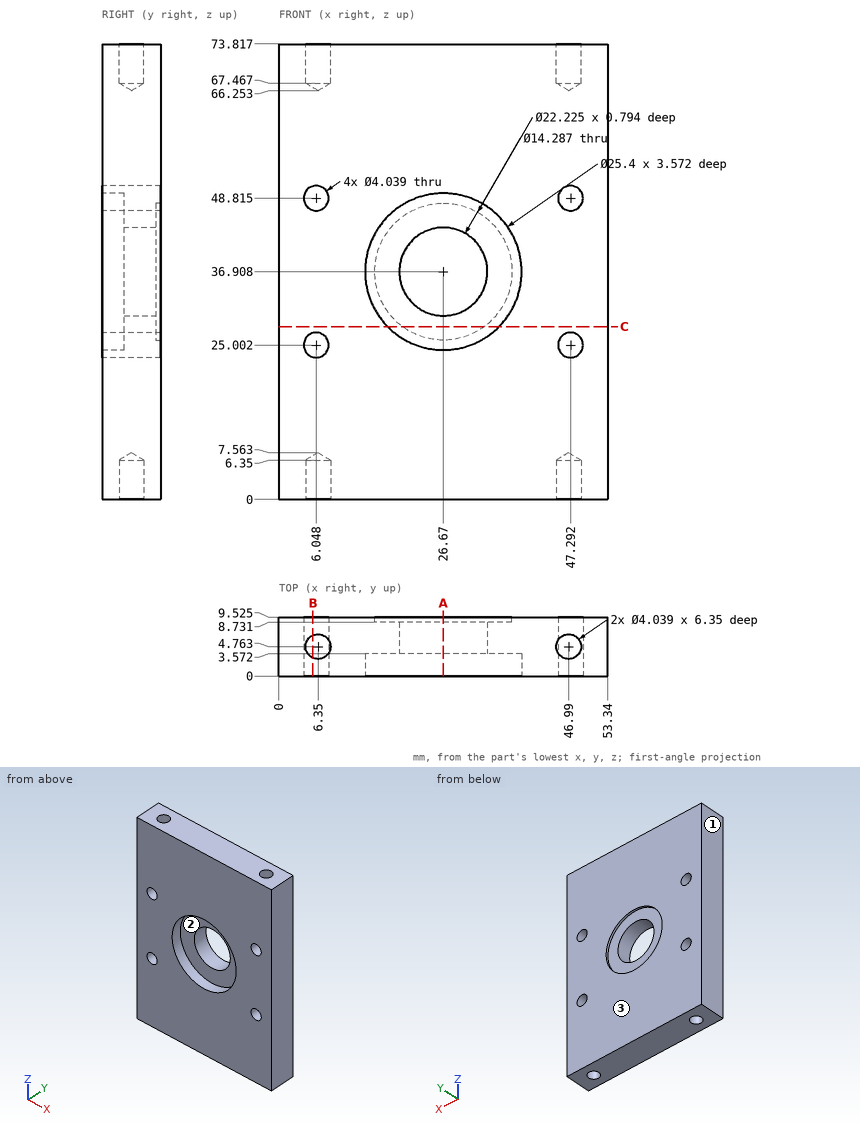
Design review of the part shown in the three views and the two pictorial views. Dimensions are in mm from the part's minimum x, y and z. Round coordinates to 2 decimals unless told otherwise and drop trailing zeros. Write each loop counter-clockwise with the first axis right and the second up, starting at its lowest first coordinate (ties: lowest second). Pieces come first, ordered by that corner, then holes. Notation, with made-up numbers: (77.5, 59.25) -> (125.5, 59.25) arc R10 ccw to (125.5, 71.25) -> close; hole circle Ø1 at (5.25, 49). An arc over 180 degrees is marked (long way). Write item = value, one per line. Start each with the question number.
1) Take a section at B-B, the plane x = 5.5. Count the separate pieces of the cut face and the enclosed holes in it.
2) Take a section at A-A, the plane x = 26.67. State the section outline as (y, z) points (1 decimal).
3) Mouldability with a two-part tool opening along X and no side actions: class the marked faces 1, 2 and 3 as +X half, -X half, draft (parallel to the pull), parting line (faces both ways), or undercut.
4) Clearance check with flat-ended pins moving along their axes: pin 1 (11 mm diameter, centred on x = 31, z = 37, fed in from +Y); pin 2 (3 mm diameter, centred on x = 6.05, z = 48.81, fed in from -Y) (3 decimals); pin 3 (3 mm diameter, centred on x = 46.99, y = 4.76, fed in from -Z); pin 4 (2.5 mm diameter, centred on x = 6.35, y = 4.76, fed in from +Z) (1 decimal). State where each tip first meets the part, or that it passes through.
5) Take a section at C-C, the plane z = 28. State the section outline as (x, y) points (1 decimal).
6) Wall thickness on probe 1 along Z at (x, y) = (30, 4) (1 decimal); probe 2 along X at (y, z) = (3.5, 29.5) (1 decimal); probe 3 along X at (y, z) = (5.5, 5.5): over which ranges is each line inside the solid? List them lowest first. Write a range as from..to.
Results list:
q1.separate_pieces = 3
q1.enclosed_holes = 0
q2.outline = (0, 0) -> (9.5, 0) -> (9.5, 25.8) -> (8.7, 25.8) -> (8.7, 29.8) -> (3.6, 29.8) -> (3.6, 24.2) -> (0, 24.2) -> close; (0, 49.6) -> (3.6, 49.6) -> (3.6, 44.1) -> (8.7, 44.1) -> (8.7, 48) -> (9.5, 48) -> (9.5, 73.8) -> (0, 73.8) -> close
q3.face_1 = -X half
q3.face_2 = undercut
q3.face_3 = draft
q4.pin_1 = 8.73
q4.pin_2 = through
q4.pin_3 = 6.66
q4.pin_4 = 67
q5.outline = (0, 0) -> (17.6, 0) -> (17.6, 3.6) -> (35.7, 3.6) -> (35.7, 0) -> (53.3, 0) -> (53.3, 9.5) -> (33.3, 9.5) -> (33.3, 8.7) -> (20, 8.7) -> (20, 9.5) -> (0, 9.5) -> close
q6.probe_1 = 0..30.6, 43.2..73.8
q6.probe_2 = 0..16.4, 37..53.3
q6.probe_3 = 0..4.47, 8.23..45.11, 48.87..53.34
